Geometry check sheet. Reference: drawing and pictorial views, mm from the part's lowest x, y, z. A direction names the side the tool comes from. Give positions to 0.01 mm unless a question says otherwise; leave off trailing zeros. Order: outer loops, then holes, each group sorted by start corner. A loop starts at its lowest first (then second) coordinate and runs counter-clockwise, first axis right, second up.
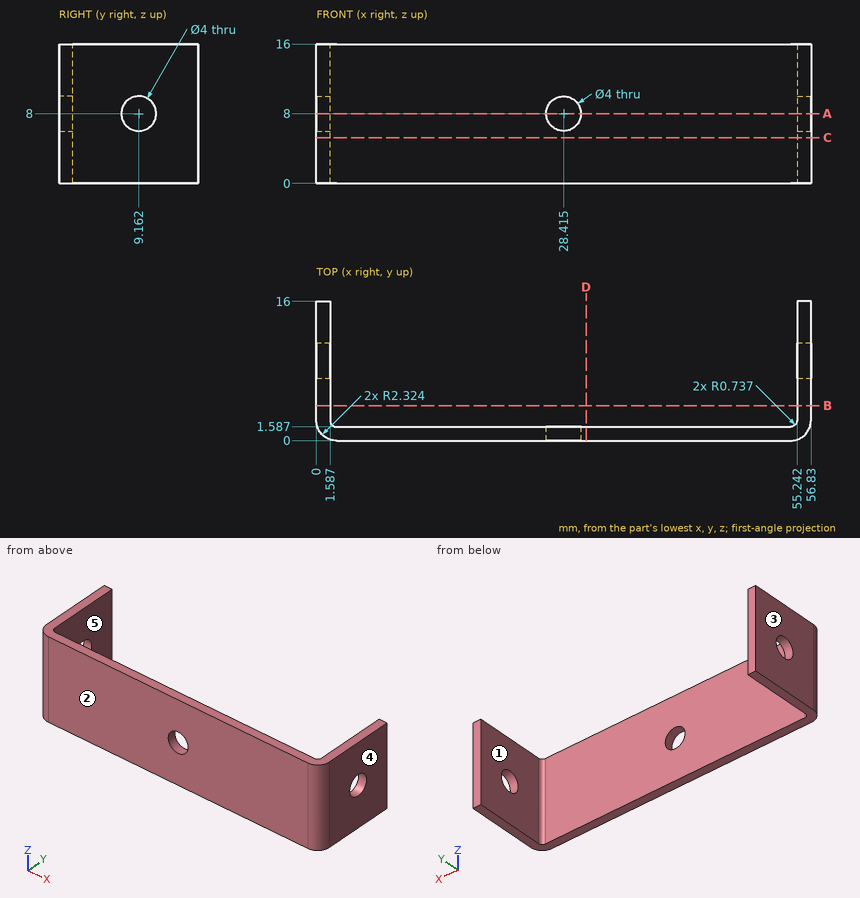
1) Section check A-A, the plane z = 8. Record the cut outline in (x, y) (1 decimal), then the cut area to 3 significant figures.
Recorded:
outline: (0, 2.3) arc R2.3 ccw to (2.3, 0) - (26.4, 0) - (26.4, 1.6) - (2.3, 1.6) arc R0.7 cw to (1.6, 2.3) - (1.6, 7.2) - (0, 7.2) - close; (0, 11.2) - (1.6, 11.2) - (1.6, 16) - (0, 16) - close; (30.4, 0) - (54.5, 0) arc R2.3 ccw to (56.8, 2.3) - (56.8, 7.2) - (55.2, 7.2) - (55.2, 2.3) arc R0.7 cw to (54.5, 1.6) - (30.4, 1.6) - close; (55.2, 11.2) - (56.8, 11.2) - (56.8, 16) - (55.2, 16) - close
area: 115 mm2
2) Set-up check for the marked faces 1 and 2: record each of +Z, -Z, +X, -X, +Y, -Y from which the full face is reachable in a straight line by a thin tool's end or side.
Recorded:
face 1: +Z, -Z, +Y
face 2: +Z, -Z, +X, -X, -Y
3) Section check D-D, the plane x = 31. Record the cut outline in (y, z).
Recorded:
outline: (0, 0) - (1.59, 0) - (1.59, 16) - (0, 16) - close
4) Section check C-C, the plane z = 5.25. Record the cut outline in (x, y) (1 decimal), then the cut area to 3 significant figures.
Recorded:
outline: (0, 2.3) arc R2.3 ccw to (2.3, 0) - (54.5, 0) arc R2.3 ccw to (56.8, 2.3) - (56.8, 16) - (55.2, 16) - (55.2, 2.3) arc R0.7 cw to (54.5, 1.6) - (2.3, 1.6) arc R0.7 cw to (1.6, 2.3) - (1.6, 16) - (0, 16) - close
area: 134 mm2
5) Draft check along X on the marked faces 3, 4 and 5. Enter one of: +X half, -X half, draft (parallel to the pull), parting line (faces both ways), or undercut.
Recorded:
face 3: -X half
face 4: +X half
face 5: undercut
6) Section check B-B, the plane y = 4. Record the cut outline in (x, z).
Recorded:
outline: (0, 0) - (1.59, 0) - (1.59, 16) - (0, 16) - close; (55.24, 0) - (56.83, 0) - (56.83, 16) - (55.24, 16) - close
7) Depth check by flat-ended pin: pin 1 Ø6.5 at (y, z) = (9.16, 8) entering from +X; pin 2 Ø4.5 at (x, z) = (28.415, 8) entering from +Y; pin 3 Ø2.5 at (y, z) = (9.16, 8) entering from -X (3 decimals). Enter the tip coordinate at first touch or a pass-through.
Recorded:
pin 1: stops at x = 56.83
pin 2: stops at y = 1.59
pin 3: passes through
8) Material ranges on L1, parallel to X at y = 11.25, z = 10; L2, parallel to X at y = 0.9, z = 8 (1 decimal); L3, parallel to Y at x = 25.5, z = 10, recorded low to high.
Recorded:
L1: x = 0 to 1.59, 55.24 to 56.83
L2: x = 0.5 to 26.4, 30.4 to 56.3
L3: y = 0 to 1.59
